```python
from build123d import *

# Parameters (mm, degrees)
SKETCH2_W           = 250
SKETCH2_H           = 250
BOSS_EXTRUDE1_DEPTH = 3.175
SKETCH3_W           = 8.6
SKETCH3_H           = 15.35
CUT_EXTRUDE1_DEPTH  = 10
SKETCH4_W           = 45.1
SKETCH4_H           = 25.1
SKETCH4_W_2         = 25.1
SKETCH4_H_2         = 45.1
CUT_EXTRUDE2_DEPTH  = 10
M3_TAPPED_HOLE1_D   = 2.5
M3_TAPPED_HOLE2_D   = 2.5
SKETCH9_R           = 0.5
CUT_EXTRUDE3_DEPTH  = 4.175


with BuildPart() as part:
    # Sketch2 → Boss-Extrude1 (new body)
    with BuildSketch(Plane(origin=(0, 0, 0), x_dir=(1, 0, 0), z_dir=(0, 1, 0))):
        Rectangle(SKETCH2_W, SKETCH2_H)
    extrude(amount=BOSS_EXTRUDE1_DEPTH)

    # Sketch3 → Cut-Extrude1 (cut)
    with BuildSketch(Plane(origin=(0, 3.175, 0), x_dir=(1, 0, 0), z_dir=(0, 1, 0))):
        with Locations((-43.75, 35.675)):
            Rectangle(SKETCH3_W, SKETCH3_H)
        with Locations((-43.75, -35.675)):
            Rectangle(SKETCH3_W, SKETCH3_H)
        with Locations((43.75, -35.675)):
            Rectangle(SKETCH3_W, SKETCH3_H)
        with Locations((43.75, 35.675)):
            Rectangle(SKETCH3_W, SKETCH3_H)
    extrude(amount=-CUT_EXTRUDE1_DEPTH, mode=Mode.SUBTRACT)

    # Sketch4 → Cut-Extrude2 (cut)
    with BuildSketch(Plane(origin=(0, 3.175, 0), x_dir=(1, 0, 0), z_dir=(0, 1, 0))):
        with Locations((0, 125)):
            Rectangle(SKETCH4_W, SKETCH4_H)
        with Locations((125, 0)):
            Rectangle(SKETCH4_W_2, SKETCH4_H_2)
        with Locations((0, -125)):
            Rectangle(SKETCH4_W, SKETCH4_H)
        with Locations((-125, 0)):
            Rectangle(SKETCH4_W_2, SKETCH4_H_2)
    extrude(amount=-CUT_EXTRUDE2_DEPTH, mode=Mode.SUBTRACT)

    # M3 Tapped Hole1 (through all)
    with Locations(Plane(origin=(0, 3.175, 0), x_dir=(1, 0, 0), z_dir=(0, 1, 0))):
        with Locations((-115, 115)):
            Hole(M3_TAPPED_HOLE1_D / 2)

    # M3 Tapped Hole2 (through all)
    with Locations(Plane(origin=(0, 3.175, 0), x_dir=(1, 0, 0), z_dir=(0, 1, 0))):
        with Locations((115, 115), (115, -115), (-115, -115)):
            Hole(M3_TAPPED_HOLE2_D / 2)

    # Sketch9 → Cut-Extrude3 (cut, through all)
    with BuildSketch(Plane(origin=(0, 3.175, 0), x_dir=(1, 0, 0), z_dir=(0, 1, 0))):
        with Locations((-92.05, -113)):
            Circle(SKETCH9_R)
        with Locations((-89.55, -114.5)):
            Circle(SKETCH9_R)
        with Locations((-59.95, -118)):
            Circle(SKETCH9_R)
        with Locations((-29.55, -118)):
            Circle(SKETCH9_R)
        with Locations((-29.55, -68)):
            Circle(SKETCH9_R)
        with Locations((-54.85, -69.6)):
            Circle(SKETCH9_R)
        with Locations((-59.95, -68)):
            Circle(SKETCH9_R)
        with Locations((-96.55, -68)):
            Circle(SKETCH9_R)
        with Locations((-93.65, -68)):
            Circle(SKETCH9_R)
        with Locations((-96.55, -71)):
            Circle(SKETCH9_R)
    extrude(amount=-CUT_EXTRUDE3_DEPTH, mode=Mode.SUBTRACT)


solid = part.part
```
Geometry check sheet. Reference: the model listing, model coordinates, mm. Coordinates: 2 decimals unless noted, no trailing zeros. Loops run counter-clockwise (first coordinate to the right, second up) from the corner with the lowest first, then second, coordinate; pieces in that order, holes last.
Item 1: Thickness scan on line 1 (Z direction, x = 42, y = 0.25); line 2 (Z direction, x = -96.55, y = 1); line 3 (Z direction, x = 114, y = 1.4). Record the ranges inside material, lowest first.
Item 2: Go/stop test with a flat-tipped pin: pin 1 Ø1.5 at (x, y) = (-20, 1) entering from -Z. Record where the tip stops, or that it passes through.
Item 3: Sectioned sample at A-A, the plane y = 2.05. Count the separate pieces of the cut face and the enclosed holes in it, then the cut area to 3 significant figures.
Item 4: Sectioned sample at B-B, the plane x = 9. Record the boundary of the cut face in (y, z) (3 decimals).
Check result:
1. line 1: z = -125 to -43.35, -28 to 28, 43.35 to 125
1. line 2: z = -125 to 67.5, 68.5 to 70.5, 71.5 to 125
1. line 3: z = -125 to -115.75, -114.25 to -22.55, 22.55 to 114.25, 115.75 to 125
2. pin 1: stops at z = -112.45
3. separate pieces: 1
3. enclosed holes: 18
3. area: 59,700 mm2
4. outline: (0, -112.45) - (3.175, -112.45) - (3.175, 112.45) - (0, 112.45) - close
